from build123d import *

# Parameters (mm, degrees)
F0_W     = 238.125
F0_H     = 168.275
F1_DEPTH = 6.35
F2_R     = 5.08
F4_DEPTH = 25.4
F6_DEPTH = 25.4
F7_R     = 0.7874


with BuildPart() as f1:
    # F0 (on Top) → F1 (new body)
    with BuildSketch(Plane.XY):
        Rectangle(F0_W, F0_H)
    extrude(amount=F1_DEPTH)

    # F2
    f2_edges = [f1.edges().sort_by_distance(p)[0] for p in [
        (119.0625, 84.1375, 3.175),
        (119.0625, -84.1375, 3.175),
        (-119.0625, -84.1375, 3.175),
        (-119.0625, 84.1375, 3.175),
    ]]
    fillet(f2_edges, radius=F2_R)

    # F3 (on face) → F4 (cut)
    with BuildSketch(Plane.XY.offset(6.35)):
        Polygon((22.479, 44.901281), (-22.479, 44.901281), (-67.380281, 0), (-22.479, -44.901281), (22.479, -44.901281), (67.380281, 0), align=None)
    extrude(amount=-F4_DEPTH, mode=Mode.SUBTRACT)

    # F5 (on face) → F6 (cut)
    with BuildSketch(Plane.XY.offset(6.35)):
        Polygon((23.005051, 46.171281), (-23.005051, 46.171281), (-69.176332, 0), (-23.005051, -46.171281), (23.005051, -46.171281), (69.176332, 0), align=None)
    extrude(amount=-F6_DEPTH, mode=Mode.SUBTRACT)

    # F7
    f7_edges = [f1.edges().sort_by_distance(p)[0] for p in [
        (-23.005051, 46.171281, 3.175),
        (23.005051, 46.171281, 3.175),
        (-69.176332, 0, 3.175),
        (-23.005051, -46.171281, 3.175),
        (23.005051, -46.171281, 3.175),
        (69.176332, 0, 3.175),
    ]]
    fillet(f7_edges, radius=F7_R)


solid = f1.part
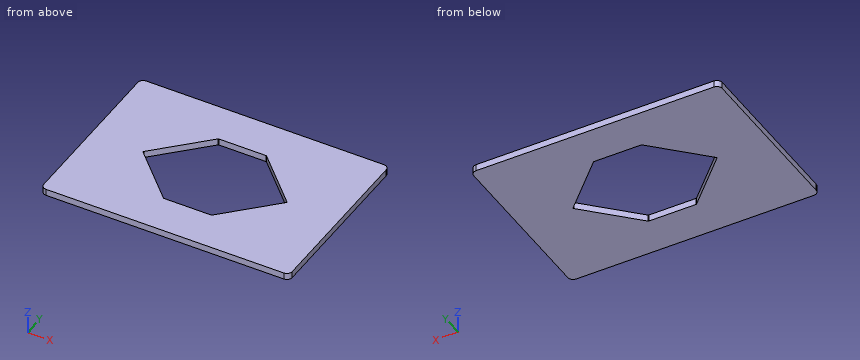
Verification items for the finished model (mm, model axes). Round coordinates to 2 decimals unless told otherwise and drop trailing zeros. Order: outer loops, then holes, each group sorted by start corner. A loop starts at its lowest first (then second) coordinate and runs counter-clockwise, first axis right, second up. Notation, with made-up numbers: (-21, -25.5) -> (12, -25.5) arc R16 cw to (12, -2.5) -> close; hole circle Ø4 at (67.25, -25). An arc over 180 degrees is marked (long way). Put each result on its own line as item: value.
1) Section check C-C (y = -14.5). Record the cut outline in (x, z).
Final values:
outline: (-119.06, 0) -> (-54.68, 0) -> (-54.68, 6.35) -> (-119.06, 6.35) -> close; (54.68, 0) -> (119.06, 0) -> (119.06, 6.35) -> (54.68, 6.35) -> close
2) Section check B-B (x = 5). Record the cut outline in (y, z), then the cut area to 3 significant figures.
Final values:
outline: (-84.14, 0) -> (-46.17, 0) -> (-46.17, 6.35) -> (-84.14, 6.35) -> close; (46.17, 0) -> (84.14, 0) -> (84.14, 6.35) -> (46.17, 6.35) -> close
area: 482 mm^2
3) Section check A-A (z = 2). Record the cut outline in (x, y), then the cut area to 3 significant figures.
Final values:
outline: (-119.06, -79.06) arc R5.08 ccw to (-113.98, -84.14) -> (113.98, -84.14) arc R5.08 ccw to (119.06, -79.06) -> (119.06, 79.06) arc R5.08 ccw to (113.98, 84.14) -> (-113.98, 84.14) arc R5.08 ccw to (-119.06, 79.06) -> close; hole (-68.62, -0.56) -> (-23.24, -45.94) arc R0.79 ccw to (-22.68, -46.17) -> (22.68, -46.17) arc R0.79 ccw to (23.24, -45.94) -> (68.62, -0.56) arc R0.79 ccw to (68.62, 0.56) -> (23.24, 45.94) arc R0.79 ccw to (22.68, 46.17) -> (-22.68, 46.17) arc R0.79 ccw to (-23.24, 45.94) -> (-68.62, 0.56) arc R0.79 ccw to start
area: 31,500 mm^2
4) Material ranges on line 1 (Y direction, x = -7.5, z = 5.5); line 2 (Y direction, x = -51, z = 6); line 3 (X direction, y = -41, z = 5.5), recorded low to high.
Final values:
line 1: y = -84.14 to -46.17, 46.17 to 84.14
line 2: y = -84.14 to -18.18, 18.18 to 84.14
line 3: x = -119.06 to -28.18, 28.18 to 119.06
